from build123d import *

# Parameters (mm, degrees)
F1_DEPTH = 280
F2_R     = 4.25
F3_DEPTH = 5.001
F4_R     = 2
F5_R     = 5
F6_R     = 4.25
F7_DEPTH = 5.001


with BuildPart() as f1:
    # F0 (on Right) → F1 (new body)
    with BuildSketch(Plane.YZ):
        Polygon((5, -92.5), (5, 87.5), (0, 87.5), (0, -87.5), (-40, -87.5), (-40, -92.5), align=None)
    extrude(amount=F1_DEPTH)

    # F2 (on face) → F3 (cut, through all)
    with BuildSketch(Plane.XZ):
        with Locations((25, 56.499322)):
            Circle(F2_R)
        with Locations((250, 56.654073)):
            Circle(F2_R)
        with Locations((250, -61.5)):
            Circle(F2_R)
        with Locations((25, -61.5)):
            Circle(F2_R)
    extrude(amount=-F3_DEPTH, mode=Mode.SUBTRACT)

    # F4
    f4_edges = [f1.edges().sort_by_distance(p)[0] for p in [
        (280, 2.5, 87.5),
        (0, 2.5, 87.5),
        (0, -40, -90),
        (280, -40, -90),
        (140, 0, -87.5),
    ]]
    fillet(f4_edges, radius=F4_R)

    # F5
    f5_edges = [f1.edges().sort_by_distance(p)[0] for p in [
        (140, 5, -92.5),
    ]]
    fillet(f5_edges, radius=F5_R)

    # F6 (on face) → F7 (cut, through all)
    with BuildSketch(Plane.XY.offset(-87.5)):
        with Locations((140, -20)):
            Circle(F6_R)
    extrude(amount=-F7_DEPTH, mode=Mode.SUBTRACT)


solid = f1.part
Model file for the job. Use its own axes, mm. A direction names the side the tool comes from. Give positions to 0.01 mm unless a question says otherwise; leave off trailing zeros. Order: outer loops, then holes, each group sorted by start corner. A loop starts at its lowest first (then second) coordinate and runs counter-clockwise, first axis right, second up. Notation, with made-up numbers: M -10,29.25 L 35,29.25 A34 ccw 35,67.25 Z; hole C -19,-19.75 d9. An arc over 180 degrees is marked long. Put each result on its own line as item: value. Start each with the question number.
(1) Pull direction X, two halves, no side cores. Call faces 1 (the face through (280, 3, -23)), 2 (the face through (136.63, -22.59, -89.96)), 3 (the face through (0, 3, -23)): released by +X, released by -X, zero draft, split by the parting line, or undercut.
(2) Band-saw the part on C-C on y = -20. Give the cut face in (x, z), then the cut area to 3 significant figures.
(3) Band-saw the part on B-B on x = 250. Give the cut face in (y, z).
(4) Drill centre lines: L1, parallel to X at y = 2, z = -61; L2, parallel to Z at x = 250, y = 2.25; L3, parallel to Z at x = 250, y = 1.7. Where is each one in solid material? Low to high. Write a range as [from, to].
(5) Band-saw the part on A-A on z = -61.5. Give the cut face in (x, y), then the cut area to 4 significant figures.
(6) Tool access for faces 4 (the face through (138, 0, 2)), 5 (the face through (138, 5, -1)): list every direction of +Z, -Z, +X, -X, +Y, -Y with a clear straight run to the whole face (end or side of a thin tool).
(7) Pin check, flat tips, straight feed: pin 1 Ø10 at (x, z) = (250, 56.65) entering from -Y; pin 2 Ø11.5 at (x, y) = (148, -21.5) entering from +Z; pin 3 Ø12 at (x, y) = (32, -7.5) entering from +Z. Stop position of each tip, or through.
(8) Band-saw the part on D-D on x = 140. Give the cut face in (y, z).
Results below:
1. face 1: released by +X
1. face 2: undercut
1. face 3: released by -X
2. outline: M 0,-92.5 L 135.75,-92.5 L 135.75,-87.5 L 0,-87.5 Z; M 144.25,-92.5 L 280,-92.5 L 280,-87.5 L 144.25,-87.5 Z
2. area: 1,360 mm2
3. outline: M -40,-92.5 L 0,-92.5 A5 ccw 5,-87.5 L 5,-65.75 L 0,-65.75 L 0,-85.5 A2 cw -2,-87.5 L -40,-87.5 Z; M 0,-57.25 L 5,-57.25 L 5,52.4 L 0,52.4 Z; M 0,60.9 L 5,60.9 L 5,87.5 L 0,87.5 Z
4. L1: x = [0, 20.78], [29.22, 245.78], [254.22, 280]
4. L2: z = [-91.97, -65.75], [-57.25, 52.4], [60.9, 87.5]
4. L3: z = [-92.2, -65.75], [-57.25, 52.4], [60.9, 87.5]
5. outline: M 0,0 L 20.75,0 L 20.75,5 L 0,5 Z; M 29.25,0 L 245.75,0 L 245.75,5 L 29.25,5 Z; M 254.25,0 L 280,0 L 280,5 L 254.25,5 Z
5. area: 1,315 mm2
6. face 4: +Z, +X, -X, -Y
6. face 5: +Z, -Z, +X, -X, +Y
7. pin 1: stops at y = 0
7. pin 2: stops at z = -87.5
7. pin 3: stops at z = -87.44
8. outline: M -40,-92.5 L -24.25,-92.5 L -24.25,-87.5 L -40,-87.5 Z; M -15.75,-92.5 L 0,-92.5 A5 ccw 5,-87.5 L 5,87.5 L 0,87.5 L 0,-85.5 A2 cw -2,-87.5 L -15.75,-87.5 Z
